Model file for the job. Use its own axes, mm. A direction names the side the tool comes from. Coordinates: 2 decimals unless noted, no trailing zeros. Write each loop counter-clockwise with the first axis right and the second up, starting at its lowest first coordinate (ties: lowest second). Pieces come first, ordered by that corner, then holes. Notation, with made-up numbers: (-33.75, 30) -> (-4.75, 30) arc R12 ccw to (-4.75, 50) -> close; hole circle Ø3 at (-28.75, -13.75). An arc over 180 degrees is marked (long way). Answer as a JSON object with one key per item and string values. Group by question number.
from build123d import *

# Parameters (mm, degrees)
F0_R     = 8
F1_DEPTH = 35
F3_DEPTH = 2


with BuildPart() as f1:
    # F0 (on Front) → F1 (new body)
    with BuildSketch(Plane.XZ):
        with BuildLine():
            Line((-62.010019, -11.999998), (28.996555, -11.999998))
            ThreePointArc((28.996555, -11.999998), (40.996553, 1e-06), (28.996555, 12))
            Line((28.996555, 12), (-62.003448, 12))
            ThreePointArc((-62.003448, 12), (-74.003447, 0.003286), (-62.010019, -11.999998))
        make_face()
        with Locations((-62.003448, 0)):
            Circle(F0_R, mode=Mode.SUBTRACT)
        with BuildLine():
            ThreePointArc((4.880946, -8), (-3.004283, 0), (4.880946, 8))
            Line((4.880946, 8), (28.996555, 8))
            ThreePointArc((28.996555, 8), (37.131105, 0), (28.996555, -8))
            Line((28.996555, -8), (4.880946, -8))
        make_face(mode=Mode.SUBTRACT)
    extrude(amount=F1_DEPTH)

    # F2 (on face) → F3 (join)
    with BuildSketch(Plane.XY.offset(12)):
        Polygon((9.892042, -14.4872), (4.819268, -11.726497), (-0.107958, -14.739297), (0.03759, -20.5128), (5.110364, -23.273503), (10.03759, -20.260703), align=None)
        Polygon((-57.003448, -20.386751), (-57.003448, -14.613249), (-62.003448, -11.726497), (-67.003448, -14.613249), (-67.003448, -20.386751), (-62.003448, -23.273503), align=None)
    extrude(amount=F3_DEPTH)


solid = f1.part
(1) 3-axis set-ups, long thin cutter, end or side, ignore diameter. For faces 5 (the face through (17, -17, 8)), 6 (the face through (7.391, -13.126, 12.986)), 7 (the face through (-67.003, -17, 13)), 8 (the face through (-57.003, -18, 13)): which of +Z, -Z, +X, -X, +Y, -Y reach the whole face in a straight line?
(2) Cut at B-B on x = 12. List the corners of the cut face in (y, z), plus the area to 3 significant figures.
(3) Cut at D-D on x = -65. List the corners of the cut face in (y, z), plus the area to 3 significant figures.
(4) Wall check: probe 1 along X at (y, z) = (-28.5, -6.25); probe 2 along X at (y, z) = (-29.5, 5.5); probe 3 along Z at (x, y) = (13, -25.5). Give the ranges that are in metal, low to high.
(5) Pin check, flat tips, straight feed: pin 1 (1.5 mm diameter, centred on x = -63.5, y = -20, fed in from -Z); pin 2 (7 mm diameter, centred on x = 21.5, y = -17, fed in from +Z); pin 3 (1.6 mm diameter, centred on y = -18, z = 13.5, fed in from -X). Stop position of each tip, or through.
(6) Pull direction X, two halves, no side cores. Call faces 1 (the face through (-64, -17, 12)), 2 (the face through (-59.54, -21.85, 12.99)), 3 (the face through (40.994, -17.255, -0.264)), 4 (the face through (-64.54, -21.81, 12.99)): released by +X, released by -X, zero draft, split by the parting line, or undercut.
(7) Cut at C-C on y = -8. List the corners of the cut face in (x, z).
(8) Cut at A-A on z = 0. List the corners of the cut face in (x, y), plus the area to 3 significant figures.
Results found:
{
 "1": {"face 5": "+Y, -Y", "face 6": "+Z, +X, +Y", "face 7": "+Z, -X, +Y, -Y", "face 8": "+Z, +Y, -Y"},
 "2": {"outline": "(-35, -12) -> (0, -12) -> (0, -8) -> (-35, -8) -> close; (-35, 8) -> (0, 8) -> (0, 12) -> (-35, 12) -> close", "area": "280 mm²"},
 "3": {"outline": "(-35, -11.62) -> (0, -11.62) -> (0, -7.42) -> (-35, -7.42) -> close; (-35, 7.42) -> (0, 7.42) -> (0, 11.62) -> (-35, 11.62) -> close; (-21.54, 12) -> (-13.46, 12) -> (-13.46, 14) -> (-21.54, 14) -> close", "area": "310 mm²"},
 "4": {"probe 1": "x = -72.25 to -67, -57.01 to 0, 34.13 to 39.24", "probe 2": "x = -72.67 to -67.81, -56.19 to -0.81, 34.94 to 39.66", "probe 3": "z = -12 to -8, 8 to 12"},
 "5": {"pin 1": "stops at z = -11.98", "pin 2": "stops at z = 12", "pin 3": "stops at x = -67"},
 "6": {"face 1": "undercut", "face 2": "undercut", "face 3": "released by +X", "face 4": "released by -X"},
 "7": {"outline": "(-62.01, -12) -> (29, -12) arc R12 ccw to (29, 12) -> (-62, 12) arc R12 ccw to start; hole circle Ø16 at (-62, 0); hole (4.88, -8) -> (29, -8) arc R8 ccw (long way) to (29, 8) -> (4.88, 8) arc R8 ccw to start"},
 "8": {"outline": "(-74, -35) -> (-70, -35) -> (-70, 0) -> (-74, 0) -> close; (-54, -35) -> (-3, -35) -> (-3, 0) -> (-54, 0) -> close; (37.13, -35) -> (41, -35) -> (41, 0) -> (37.13, 0) -> close", "area": "2,060 mm²"}
}
